Work out the finished part from the listing and answer in its coordinate system (mm). A direction names the side the tool comes from. Coordinates: 2 decimals unless noted, no trailing zeros. Write each loop counter-clockwise with the first axis right and the second up, starting at its lowest first coordinate (ties: lowest second). Pieces come first, ordered by that corner, then holes. Notation, with made-up numbers: M 43,30.25 L 66,30.25 A29 cw 66,68.25 Z; hole C 65,31.25 d10. An arc over 180 degrees is marked long. Answer as CSV lines item,"result". Start each with the question number.
(1) Flat-ended cylindrical pins translate along their axes: P1, Ø1, axis at y = 2.5, z = -3.5, coming from the +X side; P2, Ø6, axis at x = 75.5, z = -3.5, coming from the +Y side. Find the tip coordinate at first contact, or state that the pin passes through.
(2) For faces 5 (the flat face through (-2, 0, 5.563)), 6 (the cylindrical face through (52.04, 3.05, 1.26)), determine the directions among +Z, -Z, +X, -X, +Y, -Y from which every point of the face is accessible in a straight line to the end or side of a thin tool.
(3) Find the intervals of material crossed by L1, parallel to X at y = -4, z = -3.5; L2, parallel to Y at x = 83, z = 2.25; L3, parallel to Y at x = 39.5, z = 1.75, in increasing order. Write a range as [from, to].
(4) A cutting plane is placed at A-A on x = 58.5. Give the vertices of the cut face in (y, z).
(5) The mould has two halves that part along Y. Classify faces 1 (the cylindrical face through (117.23, -0.69, -3.1)), 2 (the flat face through (127, 0, 0)), 3 (the conical face through (-4.655, 2.898, 4.991)), 4 (the flat face through (-2.354, -4.795, 2.82)): released by +Y, released by -Y, zero draft, split by the parting line, or undercut.
Autodesk Inventor part; units mm, degrees
ref_plane "Work Plane1" through (1.525, 0, 0) normal (0, 0, 1) x (1, 0, 0)
ref_plane "YZ Plane" through (0, 0, 0) normal (1, 0, 0) x (0, 1, 0)
ref_plane "XZ Plane" through (0, 0, 0) normal (0, 1, 0) x (-1, 0, 0)
sketch "Sketch1" plane through (0, 0, 0) normal (0, 0, 1) x (1, 0, 0)
  line L0 (0, 5.5626) -> (0, 3.302)
  line L1 (107.95, 3.175) -> (127, 3.175)
  line L2 (127, 3.175) -> (127, 0)
  line L3 (127, 0) -> (-0.0001, 0)
  line L4 (-25.4001, 0) -> (152.4, 0)
  line L5 (-0.0001, 0) -> (-0.0001, 5.5626)
  line L6 (-0.0001, 5.5626) -> (0, 5.5626)
  line L7 (107.95, 3.175) -> (104.7749, 3.302)
  line L8 (104.7749, 3.302) -> (0, 3.302)
  line L9 (0, -1.1125) -> (0, 6.6751)
  dimension "d0" = 127
  dimension "d1" = 19.05
  dimension "d2" = 6.35
  dimension "d9" = 0.0001
  dimension "d10" = 11.1252
  dimension "d13" = 3.1751
  dimension "d14" = 6.604
revolve "Body" add sketch "Sketch1" angle 360 about axis through (127, 0, 0) along (-1, 0, 0)
sketch "Sketch2" plane through (-0.0001, 0, 0) normal (-1, 0, 0) x (0, 0, 1)
  line L0 (0, 6.4231) -> (5.5626, 3.2116)
  line L1 (5.5626, 3.2116) -> (5.5626, -3.2116)
  line L2 (5.5626, -3.2116) -> (0, -6.4231)
  line L3 (0, -6.4231) -> (-5.5626, -3.2116)
  line L4 (-5.5626, -3.2116) -> (-5.5626, 3.2116)
  line L5 (-5.5626, 3.2116) -> (0, 6.4231)
  point P0 (0, 0)
  point P1 (0, 0)
  dimension "d11" = 11.1252
extrude "Head" add sketch "Sketch2" along normal blind 4.7752
sketch "Sketch4" plane through (0, 0, 0) normal (0, 0, 1) x (1, 0, 0)
  line L0 (-4.7753, 5.5626) -> (-4.7753, 6.4231)
  line L1 (-4.7753, 6.4231) -> (-4.2785, 6.4231)
  line L2 (-4.2785, 6.4231) -> (-4.7753, 5.5626)
  line L3 (-5.7303, 0) -> (0.9549, 0)
  line L4 (-0.0001, 6.4231) -> (-4.7753, 6.4231)
  line L5 (-4.7753, 3.2116) -> (-4.7753, 6.4231)
  dimension "d5" = 30
  dimension "d19" = 11.1252
revolve "Chamfer1" cut sketch "Sketch4" angle 360 about axis through (-10, 0, 0) along (1, 0, 0)
thread "Thread"
chamfer "Chamfer2" distance 0.7791 distance2 0.7557 1 edges at (127, -3.175, 0) measured on face at (127, -0.5202, 1.1995)
ref_plane "Work Plane1" through (1.525, 0, 0) normal (0, 0, 1) x (1, 0, 0)
fillet "Fillet2" radius 0.762 1 edges at (0, -3.302, 0)
equation "\"d0\" = NLG"
equation "\"d1\" = GEL"
equation "\"d2\" = GD"
equation "\"d10\" = SD2"
equation "\"d14\" = BDM"
equation "\"d11\" = SW"
equation "\"d3\" = KOH - SD"
equation "\"d5\" = ANG1"
equation "\"d19\" = SW0"
equation "\"d63\" = R"
equation "\"d15\" = GEL"
equation "\"d6\" = -0.5 * SPD + 0.5 * GD"
equation "\"NLG\" = 127"
equation "\"GD\" = NND"
equation "\"BDM\" = 6.604"
equation "\"KOH\" = 4.7752"
equation "\"GEL\" = 19.05"
equation "\"SW\" = 11.1252"
equation "\"SW0\" = SW"
equation "\"SPD\" = GD1"
equation "\"SD2\" = SW"
equation "\"SD\" = 0"
equation "\"ANG1\" = 30deg"
equation "\"GAL\" = 3.175"
equation "\"GUL\" = 0.238 * GAL"
equation "\"R\" = 0.762"
equation "\"d62\" = -NLG - SD + GUL"
equation "\"GD1\" = 4.79184"
equation "\"THREADDIA\" = 6.35"
equation "\"TOA\" = 30deg"
equation "\"NND\" = 6.35"
equation "\"E0\" = 1.155 * SW"
properties part number "ANSI/ASME B18.2.1 - 1/4-20 UNC - 5" material "Steel, Mild"
Here are the results:
1,P1,"stops at x = 0.05"
1,P2,"stops at y = 3.26"
2,face 5,"+Z, +X, -X, +Y, -Y"
2,face 6,"+X"
3,L1,"x = [-4.78, 0]"
3,L2,"y = [-2.42, 2.42]"
3,L3,"y = [-2.8, 2.8]"
4,outline,"C 0,0 d6.6"
5,face 1,"split by the parting line"
5,face 2,"zero draft"
5,face 3,"released by +Y"
5,face 4,"released by -Y"
